Geometry check sheet. Reference: drawing and pictorial views, mm from the part's lowest x, y, z. Give positions to 0.01 mm unless a question says otherwise; leave off trailing zeros. Loops run counter-clockwise (first coordinate to the right, second up) from the corner with the lowest first, then second, coordinate; pieces in that order, holes last. Notation, with made-up numbers: (-28, 50.5) -> (28, 50.5) arc R13 cw to (28, 58.5) -> close; hole circle Ø9 at (23.5, -32.75). An arc over 180 degrees is marked (long way). Write item = value, one per line. Start each with the question number.
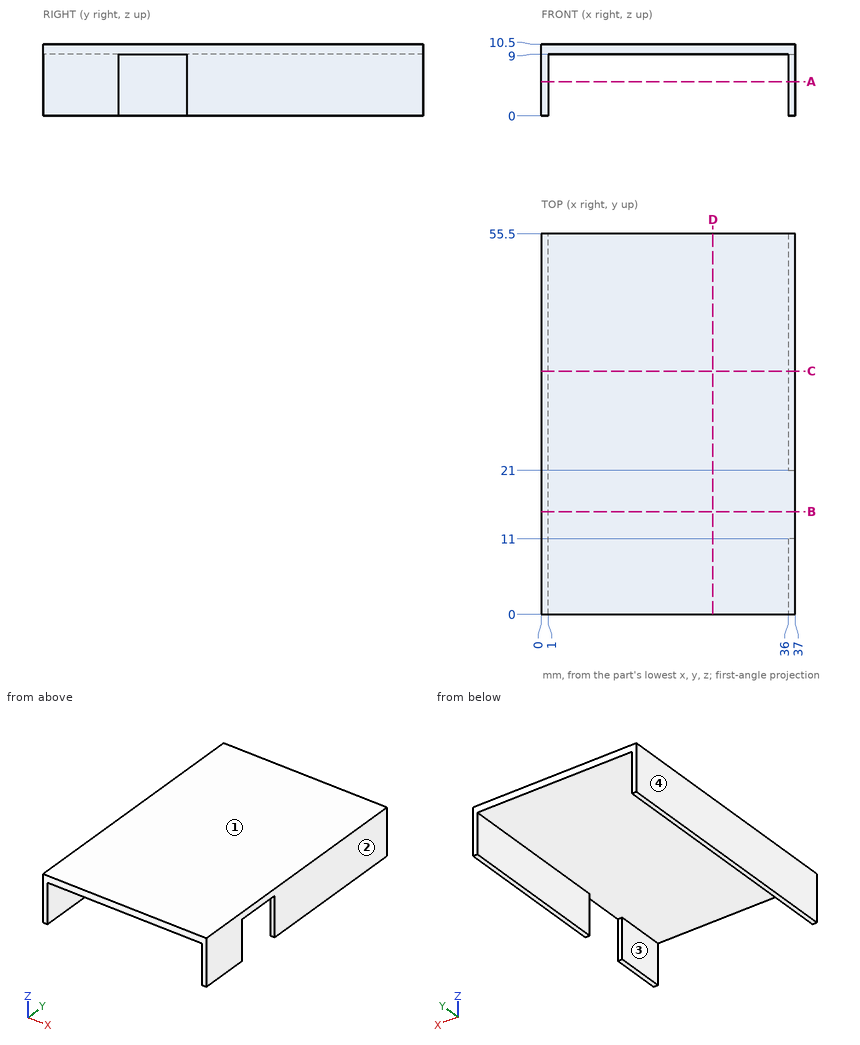
1) Depth check by flat-ended pin: pin 1 Ø1.5 at (x, y) = (20.5, 24.5) entering from -Z. Enter the tip coordinate at first touch or a pass-through.
2) Thickness scan on line 1 (X direction, y = 36.5, z = 4.75); line 2 (Z direction, x = 19.5, y = 28.5); line 3 (X direction, y = 15, z = 8). Record the ranges inside material, lowest first.
3) Section check B-B (y = 15). Enter the section's corners in (x, z).
4) Section check C-C (y = 35.5). Enter the section's corners in (x, z).
5) Section check A-A (z = 5). Enter the section's corners in (x, y), plus the area to 3 significant figures.
6) Section check D-D (x = 25). Enter the section's corners in (y, z), plus the area to 4 significant figures.
7) Draft check along X on the marked faces 1, 2, 3 and 4. Enter one of: released by +X, released by -X, zero draft, split by the parting line, or undercut.
Check result:
q1.pin_1 = 9
q2.line_1 = 0 to 1, 36 to 37
q2.line_2 = 9 to 10.5
q2.line_3 = 0 to 1
q3.outline = (0, 0) -> (1, 0) -> (1, 9) -> (37, 9) -> (37, 10.5) -> (0, 10.5) -> close
q4.outline = (0, 0) -> (1, 0) -> (1, 9) -> (36, 9) -> (36, 0) -> (37, 0) -> (37, 10.5) -> (0, 10.5) -> close
q5.outline = (0, 0) -> (1, 0) -> (1, 55.5) -> (0, 55.5) -> close; (36, 0) -> (37, 0) -> (37, 11) -> (36, 11) -> close; (36, 21) -> (37, 21) -> (37, 55.5) -> (36, 55.5) -> close
q5.area = 101 mm2
q6.outline = (0, 9) -> (55.5, 9) -> (55.5, 10.5) -> (0, 10.5) -> close
q6.area = 83.25 mm2
q7.face_1 = zero draft
q7.face_2 = released by +X
q7.face_3 = undercut
q7.face_4 = released by -X
